```python
from build123d import *

# Parameters (mm, degrees)
F0_W     = 25.4
F0_H     = 4.2683564431
F1_DEPTH = 2.54


with BuildPart() as f1:
    # F0 (on Front) → F1 (new body)
    with BuildSketch(Plane.XZ):
        Polygon((12.7, 40.6274771875), (0, 62.6245224436), (-12.7, 40.6274771875), (-25.4, 18.6304319314), (-38.1, -3.3666133248), (-50.8, -25.3636585809), (-63.5, -47.360703837), (-76.2127, -69.3797461384), (-50.8127, -69.3797461384), (-25.4127, -69.3797461384), (0, -69.3797461384), (25.4, -69.3797461384), (50.8, -69.3797461384), (76.2127, -69.3797461384), (63.50635, -47.3717023596), (50.80635, -25.3746571035), (38.10635, -3.3776118474), (25.4, 18.6304319314), align=None)
        Polygon((2.1997045256, 63.8945224436), (0, 62.6245224436), (12.7, 40.6274771875), (14.8997045256, 41.8974771875), align=None)
        Polygon((-12.7, 40.6274771875), (0, 62.6245224436), (-2.1997045256, 63.8945224436), (-14.8997045256, 41.8974771875), align=None)
        Polygon((-38.1, -3.3666133248), (-25.4, 18.6304319314), (-27.5997045256, 19.9004319314), (-40.2997045256, -2.0966133248), align=None)
        Polygon((27.5997045256, 19.9004319314), (25.4, 18.6304319314), (38.10635, -3.3776118474), (40.3060545256, -2.1076118474), align=None)
        Polygon((-63.5, -47.360703837), (-50.8, -25.3636585809), (-52.9997045256, -24.0936585809), (-65.6997045256, -46.090703837), align=None)
        Polygon((53.0060545256, -24.1046571035), (50.80635, -25.3746571035), (63.50635, -47.3717023596), (65.7060545256, -46.1017023596), align=None)
        Polygon((76.2, -73.6481025815), (76.2127, -69.3797461384), (50.8, -69.3797461384), (50.8, -73.6481025815), align=None)
        with Locations((-38.1127, -71.5139243599)):
            Rectangle(F0_W, F0_H)
        with Locations((12.7, -71.5139243599)):
            Rectangle(F0_W, F0_H)
    extrude(amount=F1_DEPTH)


solid = f1.part
```
Check sheet for the modelled part. Datum: model origin and axes. Units: mm. A direction names the side the tool comes from. Round coordinates to 2 decimals unless told otherwise and drop trailing zeros. Order: outer loops, then holes, each group sorted by start corner. A loop starts at its lowest first (then second) coordinate and runs counter-clockwise, first axis right, second up. Notation, with made-up numbers: (-40, 70.5) -> (2, 70.5) arc R17 ccw to (2, 90.5) -> close; hole circle Ø1 at (42.25, -12.5). An arc over 180 degrees is marked (long way). Use CSV: the item, a comma, the result in double quotes.
(1) Draft check along Z on faces 1 (the face through (-1, 0, -19)), 2 (the face through (-18.961, -1.252, 29.783)), 3 (the face through (34.042, -1.252, 8.742)). Enter one of: pulls with the +Z half, pulls with the -Z half, needs draft (parallel to the pull), parting line crosses it, or undercut.
Worked out:
face 1,"needs draft"
face 2,"undercut"
face 3,"pulls with the +Z half"
(2) Material ranges on line 1 along Z through (x, y) = (13, -0.25); line 2 along Z through (x, y) = (13.5, -0.8); line 3 along X through (y, z) = (-2.05, 23.5), recorded low to high. Write a range as from..to.
Worked out:
line 1,"-73.65..40.11, 40.8..45.19"
line 2,"-73.65..39.24, 41.09..44.32"
line 3,"-22.59..22.59"
(3) Tool access check on faces 4 (the face through (-59.26, -1.25, -34.94)), 5 (the face through (-69.77, -1.25, -58.22)). Record the directions out of +Z, -Z, +X, -X, +Y, -Y that give a thin tool (end or side, any length) a straight path to the whole face; none if there is none.
Worked out:
face 4,"+Z, -X, +Y, -Y"
face 5,"-X, +Y, -Y"
(4) Cross-section at B-B (x = -42). Record the boundary of the cut face in (y, z).
Worked out:
outline,"(-2.54, -73.65) -> (0, -73.65) -> (0, -10.12) -> (-2.54, -10.12) -> close"
(5) Cross-section at A-A (z = -7). Record the boundary of the cut face in (x, y).
Worked out:
outline,"(-40.2, -2.54) -> (40.2, -2.54) -> (40.2, 0) -> (-40.2, 0) -> close"
(6) Depth check by flat-ended pin: pin 1 (1.3 mm diameter, centred on y = -1.5, z = -71, fed in from +X); pin 2 (1.5 mm diameter, centred on y = -1.5, z = -34, fed in from +X); pin 3 (1.3 mm diameter, centred on x = 42.5, y = -1.5, fed in from -Z). Enter the tip coordinate at first touch or a pass-through.
Worked out:
pin 1,"x = 76.21"
pin 2,"x = 59.15"
pin 3,"z = -69.38"
